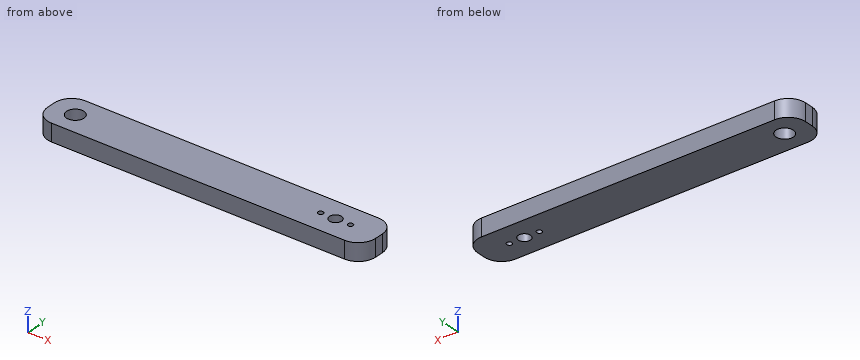
```python
from build123d import *

# Parameters (mm, degrees)
SKETCH1_R           = 5
SKETCH1_R_2         = 3.5
SKETCH1_R_3         = 1.5
BOSS_EXTRUDE1_DEPTH = 10


with BuildPart() as part:
    # Sketch1 → Boss-Extrude1 (new body)
    with BuildSketch(Plane.XY):
        with BuildLine():
            Line((0, 0), (-90.847457627, 0))
            ThreePointArc((-90.847457627, 0), (-97.918525439, -2.928932188), (-100.847457627, -10))
            Line((-100.847457627, -10), (-100.847457627, -15))
            ThreePointArc((-100.847457627, -15), (-97.918525439, -22.071067812), (-90.847457627, -25))
            Line((-90.847457627, -25), (78.152542373, -25))
            ThreePointArc((78.152542373, -25), (85.223610185, -22.071067812), (88.152542373, -15))
            Line((88.152542373, -15), (88.152542373, -10))
            ThreePointArc((88.152542373, -10), (85.223610185, -2.928932188), (78.152542373, 0))
            Line((78.152542373, 0), (0, 0))
        make_face()
        with Locations((-86.847457627, -12.5)):
            Circle(SKETCH1_R, mode=Mode.SUBTRACT)
        with Locations((63.152542373, -12.5)):
            Circle(SKETCH1_R_2, mode=Mode.SUBTRACT)
        with Locations((54.522542373, -12.5)):
            Circle(SKETCH1_R_3, mode=Mode.SUBTRACT)
        with Locations((71.782542373, -12.5)):
            Circle(SKETCH1_R_3, mode=Mode.SUBTRACT)
    extrude(amount=BOSS_EXTRUDE1_DEPTH)


solid = part.part
```
Verification items for the finished model (mm, model axes). Round coordinates to 2 decimals unless told otherwise and drop trailing zeros. Loops run counter-clockwise (first coordinate to the right, second up) from the corner with the lowest first, then second, coordinate; pieces in that order, holes last. Notation, with made-up numbers: (-17.75, 47) -> (17.25, 47) arc R25 cw to (17.25, 75) -> close; hole circle Ø6 at (81, 14). An arc over 180 degrees is marked (long way). Answer as a JSON object with one key per item and string values.
Q1. Section check A-A (z = 3.75). Record the boundary of the cut face in (x, y), then the cut area to 3 significant figures.
Data:
{"outline": "(-100.85, -15) arc R10 ccw to (-90.85, -25) -> (78.15, -25) arc R10 ccw to (88.15, -15) -> (88.15, -10) arc R10 ccw to (78.15, 0) -> (-90.85, 0) arc R10 ccw to (-100.85, -10) -> close; hole circle Ø10 at (-86.85, -12.5); hole circle Ø3 at (54.52, -12.5); hole circle Ø7 at (63.15, -12.5); hole circle Ø3 at (71.78, -12.5)", "area": "4,510 mm2"}
Q2. Scan lines: line 1 (X direction, y = -12.75, z = 7.75); line 2 (Y direction, x = 63, z = 1.5); line 3 (X direction, y = -13, z = 2.25). Record each from-to range of solid material in increasing order. Write a range as from..to.
Data:
{"line 1": "x = -100.85..-91.84, -81.85..53.04, 56..59.66, 66.64..70.3, 73.26..88.15", "line 2": "y = -25..-16, -9..0", "line 3": "x = -100.85..-91.82, -81.87..53.11, 55.94..59.69, 66.62..70.37, 73.2..88.15"}
Q3. Section check D-D (y = -22.75). Record the boundary of the cut face in (x, z).
Data:
{"outline": "(-97.17, 0) -> (84.47, 0) -> (84.47, 10) -> (-97.17, 10) -> close"}
Q4. Go/stop test with flat-tipped pins: P1, Ø2, axis at y = -3.5, z = 2, coming from the -X side; P2, Ø1, axis at x = -77, y = -13.5, coming from the -Z side; P3, Ø2, axis at y = -17.5, z = 8, coming from the -X side. Record where each tip stops, or that it passes through.
Data:
{"P1": "stops at x = -99.2", "P2": "stops at z = 0", "P3": "stops at x = -100.73"}
Q5. Section check B-B (x = -86.5). Record the boundary of the cut face in (y, z).
Data:
{"outline": "(-25, 0) -> (-17.49, 0) -> (-17.49, 10) -> (-25, 10) -> close; (-7.51, 0) -> (0, 0) -> (0, 10) -> (-7.51, 10) -> close"}
Q6. Section check C-C (x = 63). Record the boundary of the cut face in (y, z).
Data:
{"outline": "(-25, 0) -> (-16, 0) -> (-16, 10) -> (-25, 10) -> close; (-9, 0) -> (0, 0) -> (0, 10) -> (-9, 10) -> close"}
